Check sheet for the drawn part. Datum: minimum x, y, z corner. Units: mm. A direction names the side the tool comes from. Give positions to 0.01 mm unless a question says otherwise; leave off trailing zeros. Order: outer loops, then holes, each group sorted by start corner. A loop starts at its lowest first (then second) coordinate and runs counter-clockwise, first axis right, second up. Notation, with made-up numbers: (52.25, 41) -> (75.25, 41) arc R14 ccw to (75.25, 60) -> close; hole circle Ø2 at (29.25, -24). An arc over 180 degrees is marked (long way). One line per question, with ' | ' between items. Start each with the question number.
Q1. Section check C-C on y = 25.5. Record the cut outline in (x, z) (1 decimal), plus the area to 3 significant figures.
Q2. Mould release check, pull along Y, two halves, no side actions. Record for the marked faces 1, 2 and 3: released by +Y, released by -Y, zero draft, split by the parting line, or undercut.
Q3. Access from +Z, -Z, +X, -X, +Y, -Y to the whole of each face (thin tool, end or side, straight path). Record for the marked faces 4 and 5.
Q4. Section check A-A on x = 5. Give the number of separate pieces and of enclosed holes in the cut face, plus the area to 3 significant figures.
Q5. Material ranges on probe 1 along X at (y, z) = (70.5, 12.5); probe 2 along X at (y, z) = (8.5, 34) (1 decimal), recorded low to high. Write a range as [from, to].
Q6. Go/stop test with flat-tipped pins: pin 1 (19.5 mm diameter, centred on y = 28.5, z = 11, fed in from +X); pin 2 (10 mm diameter, centred on y = 73, z = 21.5, fed in from +X); pin 3 (5.5 mm diameter, centred on y = 63.5, z = 14.5, fed in from +X); pin 4 (4 mm diameter, centred on x = 11, z = 25, fed in from -Y). Record where each tip stops, or that it passes through.
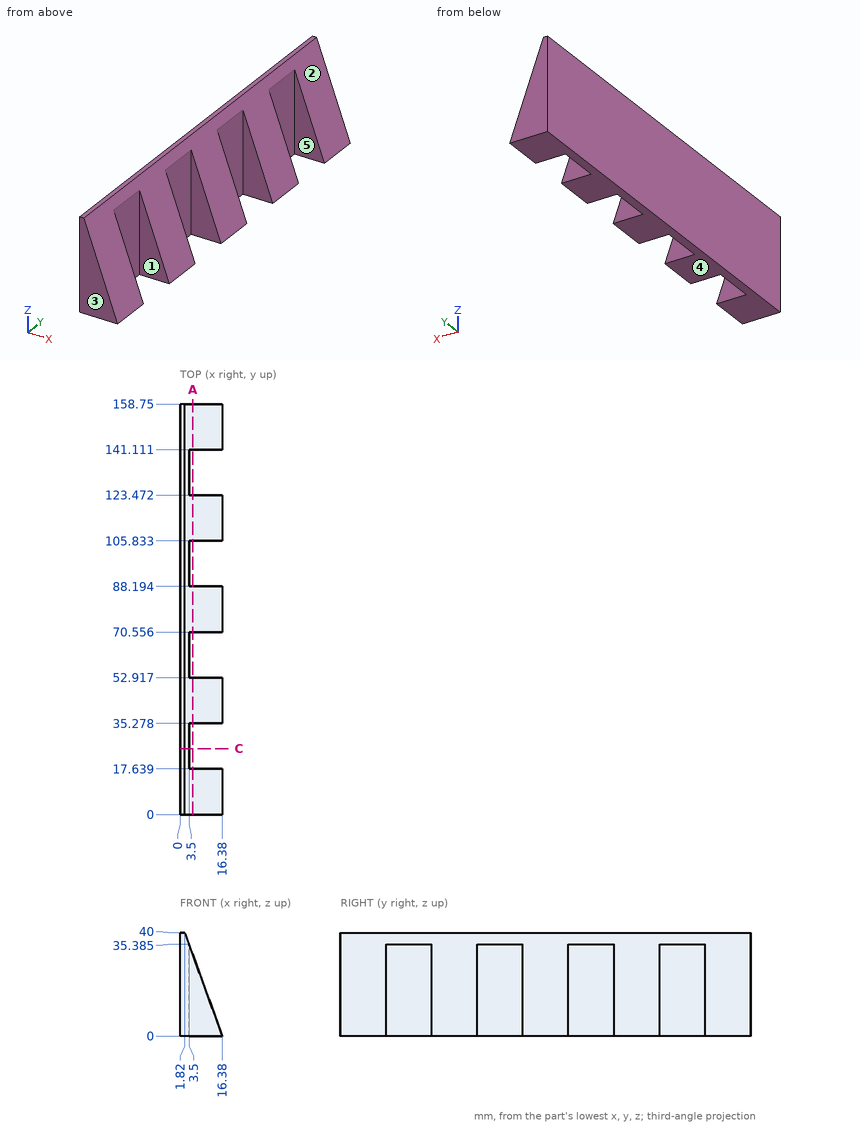
Filled in:
1) outline: (0, 0) -> (3.5, 0) -> (3.5, 35.4) -> (1.8, 40) -> (0, 40) -> close | area: 136 mm²
2) face 1: undercut | face 2: zero draft | face 3: released by -Y
3) face 4: -Z, +X, -X, +Y, -Y | face 5: +Z, -Z, +X
4) separate pieces: 5 | enclosed holes: 0 | area: 2,760 mm²
5) probe 1: [0, 3.5] | probe 2: [0, 4]
6) pin 1: x = 14.93 | pin 2: x = 10.37 | pin 3: x = 3.5 | pin 4: through
